The listing builds one solid part. Answer for the finished solid, in the listing's coordinates (mm). A direction names the side the tool comes from. Coordinates: 2 decimals unless noted, no trailing zeros. Order: outer loops, then holes, each group sorted by start corner. A loop starts at its lowest first (then second) coordinate and runs counter-clockwise, first axis right, second up. Notation, with made-up numbers: (-39.5, -25.5) -> (-3.5, -25.5) arc R19 ccw to (-3.5, 6.5) -> close; hole circle Ø1 at (-20.5, 2). An arc over 180 degrees is marked (long way). Put each result on its own line as item: value. Start each with the question number.
```python
from build123d import *

# Parameters (mm, degrees)
F1_DEPTH = 9
F2_R     = 5
F3_R     = 7.4
F5_START = -10
F5_DEPTH = 20
F7_DEPTH = 15
F8_R     = 5


with BuildPart() as f1:
    # F0 (on Top) → F1 (new body, symmetric)
    with BuildSketch(Plane.XY):
        with BuildLine():
            Line((-5, 0), (-2.4, -9.7033320997))
            Line((-2.4, -9.7033320997), (-2.4, -129.5))
            ThreePointArc((-2.4, -129.5), (-9.5872847082, -137.4586113019), (-18.2348734636, -131.1170212766))
            ThreePointArc((-18.2348734636, -131.1170212766), (-19.7482014958, -130.0072430222), (-21.0059763198, -131.4))
            ThreePointArc((-21.0059763198, -131.4), (-15.1073180305, -145.995204112), (-0.7241308269, -152.3934912697))
            ThreePointArc((-0.7241308269, -152.3934912697), (-0.2136316102, -152.1973413167), (0, -151.6939073197))
            Line((0, -151.6939073197), (0, -9.3873661055))
            Line((0, -9.3873661055), (-2.6, 0.3159659942))
            Line((-2.6, 0.3159659942), (-2.6, 12))
            Line((-2.6, 12), (-5, 12))
            Line((-5, 12), (-5, 0))
        make_face()
    extrude(amount=F1_DEPTH, both=True)

    # F2
    f2_edges = [f1.edges().sort_by_distance(p)[0] for p in [
        (-2.4, -9.703332, 0),
        (-2.6, 0.315966, 0),
    ]]
    fillet(f2_edges, radius=F2_R)

    # F3
    f3_edges = [f1.edges().sort_by_distance(p)[0] for p in [
        (-5, 0, 0),
        (0, -9.387366, 0),
    ]]
    fillet(f3_edges, radius=F3_R)

    # F4 (on Right) → F5 (cut)
    with BuildSketch(Plane.YZ.offset(F5_START)):
        with BuildLine():
            ThreePointArc((-129.4, -5), (-130.5715728753, -7.8284271247), (-133.4, -9))
            Line((-133.4, -9), (-133.4, -10))
            Line((-133.4, -10), (-128.4, -10))
            Line((-128.4, -10), (-128.4, 10))
            Line((-128.4, 10), (-133.4, 10))
            Line((-133.4, 10), (-133.4, 9))
            ThreePointArc((-133.4, 9), (-130.5715728753, 7.8284271247), (-129.4, 5))
            Line((-129.4, 5), (-129.4, -5))
        make_face()
    extrude(amount=-F5_DEPTH, mode=Mode.SUBTRACT)

    # F6 (on Right) → F7 (cut)
    with BuildSketch(Plane.YZ):
        with BuildLine():
            ThreePointArc((5.5, -5.25), (5.8535533906, -5.1035533906), (6, -4.75))
            Line((6, -4.75), (6, 4.75))
            ThreePointArc((6, 4.75), (5.8535533906, 5.1035533906), (5.5, 5.25))
            Line((5.5, 5.25), (-1, 5.25))
            ThreePointArc((-1, 5.25), (-1.7071067812, 4.9571067812), (-2, 4.25))
            Line((-2, 4.25), (-2, -4.25))
            ThreePointArc((-2, -4.25), (-1.7071067812, -4.9571067812), (-1, -5.25))
            Line((-1, -5.25), (5.5, -5.25))
        make_face()
    extrude(amount=-F7_DEPTH, mode=Mode.SUBTRACT)

    # F8
    f8_edges = [f1.edges().sort_by_distance(p)[0] for p in [
        (-3.8, 12, -9),
        (-3.8, 12, 9),
    ]]
    fillet(f8_edges, radius=F8_R)


solid = f1.part
```
(1) The part is cut by section A-A on z = 1.25. Determine the outline of the cut face in (x, y), plus the area to 3 significant figures.
(2) Find the intervals of material crossed by L1, parallel to X at y = -81.5, z = -7; L2, parallel to X at y = -136.5, z = -3; L3, parallel to X at y = 4.5, z = -7, in increasing order.
(3) The part is cut by section C-C on x = -11.5. Determine the outline of the cut face in (y, z).
(4) Each of these flat-tipped pins is pushed along its axis until it touches: P1, Ø1.2, axis at x = -3.5, z = 0, coming from the -Y side; P2, Ø1, axis at x = -2.5, z = -4.5, coming from the +Y side; P3, Ø10, axis at x = -14, z = 4.5, coming from the -Y side; P4, Ø9, axis at y = 4, z = -1.5, coming from the +X side. Where does it stop, or does it pass through?
(5) The part is cut by section B-B on y = -89.5. Determine the outline of the cut face in (x, z), plus the area to 3 significant figures.
(6) For a pull along Y with two mould halves and no side action, classify faces 1 (the cylindrical face through (-9.42, -137.44, 0.13)), 2 (the cylindrical face through (-19.57, -131.83, -8.68)), 3 (the flat face through (-4, 2, 5.25)), 4 (the flat face through (-2, -96, 9)) as released by +Y, released by -Y, zero draft, split by the parting line, or undercut.
(7) A tool of negligible diameter and unlimited length cuts with its end or side. For faces 5 (the flat face through (-2.6, 8, 0)), 6 (the flat face through (-5, 8, 0)), 7 (the flat face through (-4, 2, -5.25)), 8 (the cylindrical face through (-19.572, -131.887, 8.703)), from which of +Z, -Z, +X, -X, +Y, -Y can it reach the whole face along a straight path? Write none if from no direction.
Worked out:
1. outline: (-21.01, -131.4) arc R21.01 ccw to (-0.72, -152.39) arc R0.7 ccw to (0, -151.69) -> (0, -10.36) arc R7.4 ccw to (-0.25, -8.45) -> (-1.98, -2) -> (-4.46, -2) -> (-2.57, -9.07) arc R5 cw to (-2.4, -10.36) -> (-2.4, -129.5) arc R8 cw to (-18.23, -131.12) arc R1.4 ccw to start; (-5, 6) -> (-2.6, 6) -> (-2.6, 12) -> (-5, 12) -> close
1. area: 605 mm2
2. L1: -2.4 to 0
2. L2: -20.38 to -14.27, -6.53 to 0
2. L3: -5 to -2.6
3. outline: (-148.98, -9) -> (-137.42, -9) -> (-137.42, 9) -> (-148.98, 9) -> close
4. P1: y = -152.2
4. P2: y = 12
4. P3: y = -150.38
4. P4: x = -2.6
5. outline: (-2.4, -9) -> (0, -9) -> (0, 9) -> (-2.4, 9) -> close
5. area: 43.2 mm2
6. face 1: undercut
6. face 2: released by +Y
6. face 3: undercut
6. face 4: zero draft
7. face 5: +Z, -Z, +X, +Y
7. face 6: +Z, -Z, -X, +Y
7. face 7: +X, -X
7. face 8: +Z, -X, +Y
